```python
from build123d import *

# Parameters (mm, degrees)
BOSS_EXTRUDE1_DEPTH            = 10
CBORE_FOR_M4_SHCS1_D           = 4.5
CBORE_FOR_M4_SHCS1_CBORE_D     = 8
CBORE_FOR_M4_SHCS1_CBORE_DEPTH = 4
CBORE_FOR_M4_SHCS2_D           = 4.5
CBORE_FOR_M4_SHCS2_CBORE_D     = 8
CBORE_FOR_M4_SHCS2_CBORE_DEPTH = 4
SKETCH8_R                      = 5
BOSS_EXTRUDE2_DEPTH            = 15
FILLET1_R                      = 3
SKETCH10_R                     = 2.25
BOSS_EXTRUDE3_DEPTH            = 11.5


with BuildPart() as part:
    # Sketch1 → Boss-Extrude1 (new body)
    with BuildSketch(Plane(origin=(0, 0, 0), x_dir=(1, 0, 0), z_dir=(0, 1, 0))):
        with BuildLine():
            Line((-52.5, -16.393596311), (-52.5, 16.393596311))
            ThreePointArc((-52.5, 16.393596311), (0, 55), (52.5, 16.393596311))
            Line((52.5, 16.393596311), (52.5, -16.393596311))
            ThreePointArc((52.5, -16.393596311), (0, -55), (-52.5, -16.393596311))
        make_face()
    extrude(amount=BOSS_EXTRUDE1_DEPTH)

    # CBORE for M4 SHCS1 (through all)
    with Locations(Plane(origin=(0, 10, 0), x_dir=(1, 0, 0), z_dir=(0, 1, 0))):
        with Locations((-45, 0), (0, 45), (45, 0), (0, -45)):
            CounterBoreHole(CBORE_FOR_M4_SHCS1_D / 2, CBORE_FOR_M4_SHCS1_CBORE_D / 2, CBORE_FOR_M4_SHCS1_CBORE_DEPTH)

    # CBORE for M4 SHCS2 (through all)
    with Locations(Plane(origin=(0, 0, 0), x_dir=(-1, 0, 0), z_dir=(0, -1, 0))):
        with Locations((15, -32.5), (-15, -32.5), (15, 32.5), (-15, 32.5)):
            CounterBoreHole(CBORE_FOR_M4_SHCS2_D / 2, CBORE_FOR_M4_SHCS2_CBORE_D / 2, CBORE_FOR_M4_SHCS2_CBORE_DEPTH)

    # Sketch8 → Boss-Extrude2 (add)
    with BuildSketch(Plane(origin=(0, 10, 0), x_dir=(1, 0, 0), z_dir=(0, 1, 0))):
        with Locations((-15, 32.5)):
            Circle(SKETCH8_R)
        Polygon((-11.24722325, 32.5), (-13.123611625, 35.75), (-16.876388375, 35.75), (-18.75277675, 32.5), (-16.876388375, 29.25), (-13.123611625, 29.25), align=None, mode=Mode.SUBTRACT)
        with Locations((15, 32.5)):
            Circle(SKETCH8_R)
        Polygon((13.123611625, 29.25), (11.24722325, 32.5), (13.123611625, 35.75), (16.876388375, 35.75), (18.75277675, 32.5), (16.876388375, 29.25), align=None, mode=Mode.SUBTRACT)
        with Locations((-15, -32.5)):
            Circle(SKETCH8_R)
        Polygon((-13.123611625, -29.25), (-11.24722325, -32.5), (-13.123611625, -35.75), (-16.876388375, -35.75), (-18.75277675, -32.5), (-16.876388375, -29.25), align=None, mode=Mode.SUBTRACT)
        with Locations((15, -32.5)):
            Circle(SKETCH8_R)
        Polygon((16.876388375, -29.25), (13.123611625, -29.25), (11.24722325, -32.5), (13.123611625, -35.75), (16.876388375, -35.75), (18.75277675, -32.5), align=None, mode=Mode.SUBTRACT)
    extrude(amount=BOSS_EXTRUDE2_DEPTH)

    # Fillet1
    fillet1_edges = [part.edges().sort_by_distance(p)[0] for p in [
        (-20, 10, 32.5),
        (10, 10, 32.5),
        (-20, 10, -32.5),
        (10, 10, -32.5),
    ]]
    fillet(fillet1_edges, radius=FILLET1_R)

    # Sketch10 → Boss-Extrude3 (add)
    with BuildSketch(Plane(origin=(0, 10, 0), x_dir=(1, 0, 0), z_dir=(0, 1, 0))):
        Polygon((-13.123611625, 35.75), (-16.876388375, 35.75), (-18.75277675, 32.5), (-16.876388375, 29.25), (-13.123611625, 29.25), (-11.24722325, 32.5), align=None)
        with Locations((-15, 32.5)):
            Circle(SKETCH10_R, mode=Mode.SUBTRACT)
        Polygon((11.24722325, 32.5), (13.123611625, 35.75), (16.876388375, 35.75), (18.75277675, 32.5), (16.876388375, 29.25), (13.123611625, 29.25), align=None)
        with Locations((15, 32.5)):
            Circle(SKETCH10_R, mode=Mode.SUBTRACT)
        Polygon((13.123611625, -29.25), (11.24722325, -32.5), (13.123611625, -35.75), (16.876388375, -35.75), (18.75277675, -32.5), (16.876388375, -29.25), align=None)
        with Locations((15, -32.5)):
            Circle(SKETCH10_R, mode=Mode.SUBTRACT)
        Polygon((-11.24722325, -32.5), (-13.123611625, -35.75), (-16.876388375, -35.75), (-18.75277675, -32.5), (-16.876388375, -29.25), (-13.123611625, -29.25), align=None)
        with Locations((-15, -32.5)):
            Circle(SKETCH10_R, mode=Mode.SUBTRACT)
    extrude(amount=BOSS_EXTRUDE3_DEPTH)


solid = part.part
```
Source: CAD feature listing. Evaluate the final solid. Frame: model axes, mm. A direction names the side the tool comes from. Give positions to 0.01 mm unless a question says otherwise; leave off trailing zeros. Order: outer loops, then holes, each group sorted by start corner. A loop starts at its lowest first (then second) coordinate and runs counter-clockwise, first axis right, second up.
(1) Section query B-B (x = 1). Return the cut outline in (y, z), plus the area to 3 significant figures.
(2) Section query C-C (x = -45). Return the cut outline in (y, z), plus the area to 3 significant figures.
(3) Access query for faces 1 (the face through (13, 4, 34)), 2 (the face through (-15, 23, 35.75)), 3 (the face through (1, 0, -1)). Directions: +Z, -Z, +X, -X, +Y, -Y. A direction counts if a zero-diameter tool reaches every point of the face in a straight line with its end or side. Return the directions, or none.
(4) Section query D-D (z = -14). Return the cut outline in (x, y).
(5) Contact query for flat-ended pins moving along their axis: P1, Ø1, axis at y = 19.5, z = 26, coming from the -X side; P2, Ø6.5, axis at x = 45, z = 1, coming from the +Y side; P3, Ø1.5, axis at y = 17, z = 37.5, coming from the +X side; P4, Ø3, axis at x = 15, y = 22.5, coming from the +Z side. Output: stop coordinate, or through.
(6) Material intervals for line 1 along X through (y, z) = (16.5, -32.5); line 2 along Z through (x, y) = (-15, 2.55); line 3 along Y through (x, z) = (-10.5, -18.5), sorted ascending.
(7) Section query A-A (y = 19.5). Return the cut outline in (x, z), plus the area to 3 significant figures.
Outcome:
1. outline: (0, -54.99) - (10, -54.99) - (10, -48.87) - (6, -48.87) - (6, -47.02) - (0, -47.02) - close; (0, -42.98) - (6, -42.98) - (6, -41.13) - (10, -41.13) - (10, 41.13) - (6, 41.13) - (6, 42.98) - (0, 42.98) - close; (0, 47.02) - (6, 47.02) - (6, 48.87) - (10, 48.87) - (10, 54.99) - (0, 54.99) - close
1. area: 989 mm2
2. outline: (0, -31.62) - (10, -31.62) - (10, -4) - (6, -4) - (6, -2.25) - (0, -2.25) - close; (0, 2.25) - (6, 2.25) - (6, 4) - (10, 4) - (10, 31.62) - (0, 31.62) - close
2. area: 573 mm2
3. face 1: -Y
3. face 2: +Y
3. face 3: +Z, -Z, +X, -X, -Y
4. outline: (-52.5, 0) - (52.5, 0) - (52.5, 10) - (-52.5, 10) - close
5. P1: passes through
5. P2: stops at y = 10
5. P3: stops at x = 17.63
5. P4: stops at z = 37.5
6. line 1: x = -20 to -17.25, -12.75 to -10, 10 to 12.75, 17.25 to 20
6. line 2: z = -52.92 to -36.5, -28.5 to 28.5, 36.5 to 52.92
6. line 3: y = 0 to 10
7. outline: circle Ø10 at (-15, -32.5); circle Ø10 at (-15, 32.5); circle Ø10 at (15, -32.5); circle Ø10 at (15, 32.5); hole circle Ø4.5 at (-15, -32.5); hole circle Ø4.5 at (-15, 32.5); hole circle Ø4.5 at (15, -32.5); hole circle Ø4.5 at (15, 32.5)
7. area: 251 mm2
